Part model, mm, in its own coordinate system. Face numbers are marked on the shaded views. A direction names the side the tool comes from. Give positions to 0.01 mm unless a question says otherwise; leave off trailing zeros. Write each loop counter-clockwise with the first axis right and the second up, starting at its lowest first coordinate (ties: lowest second). Pieces come first, ordered by that corner, then holes. Notation, with made-up numbers: (-17, 85) - (25, 85) arc R23 cw to (25, 100) - close; hole circle Ø4 at (-13, 30.25). An arc over 180 degrees is marked (long way). Answer as a JSON object with one key per item and string values. Group by question number.
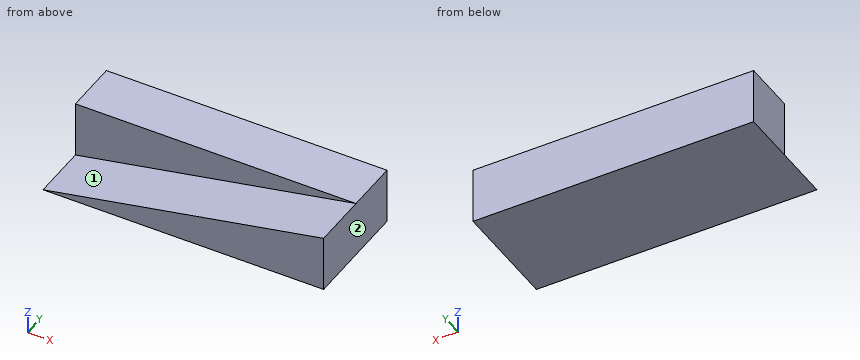
```python
from build123d import *

# Parameters (mm, degrees)
F0_W     = 126.529091
F0_H     = 49.704478
F1_DEPTH = 25.4
F3_DEPTH = 25.4


with BuildPart() as f1:
    # F0 (on Top) → F1 (new body)
    with BuildSketch(Plane.XY):
        with Locations((-4.691902, -11.49794)):
            Rectangle(F0_W, F0_H)
    extrude(amount=F1_DEPTH)

    # F2 (on face) → F3 (cut)
    with BuildSketch(Plane.XZ.offset(36.350179)):
        Polygon((-67.956448, 0), (58.572643, 25.4), (-67.956448, 25.4), align=None)
    extrude(amount=-F3_DEPTH, mode=Mode.SUBTRACT)


solid = f1.part
```
1) Saw through at B-B (z = 23.75). List the corners of the cut face in (x, y).
2) Drill centre lines: line 1 along Y through (x, z) = (-3.5, 18.75); line 2 along Z through (x, y) = (-31, -16); line 3 along Z through (x, y) = (33, -24). Where is each one in solid material? Low to high. Write a range as from..to.
3) Drop flat-ended pins along their axis: P1, Ø6, axis at x = -3.5, z = 22.5, coming from the -Y side; P2, Ø4, axis at x = -46.5, y = -26, coming from the +Z side. Give the stop position or say it passes through.
4) Which spindle directions (+Z, -Z, +X, -X, +Y, -Y) get a long thin tool onto all of the face, cutting with end or side? Do the marked faces 1 and 2. Say none if no direction does.
5) Saw through at C-C (x = 36). List the corners of the cut face in (y, z).
6) Saw through at A-A (y = -27). List the corners of the cut face in (x, z), and give its area (3 significant figures).
Checks:
{
 "1": {"outline": "(-67.96, -10.95) - (50.35, -10.95) - (50.35, -36.35) - (58.57, -36.35) - (58.57, 13.35) - (-67.96, 13.35) - close"},
 "2": {"line 1": "-10.95..13.35", "line 2": "0..7.42", "line 3": "0..20.27"},
 "3": {"P1": "y = -10.95", "P2": "z = 4.71"},
 "4": {"face 1": "+Z, -X, -Y", "face 2": "+Z, -Z, +X, +Y, -Y"},
 "5": {"outline": "(-36.35, 0) - (13.35, 0) - (13.35, 25.4) - (-10.95, 25.4) - (-10.95, 20.87) - (-36.35, 20.87) - close"},
 "6": {"outline": "(-67.96, 0) - (58.57, 0) - (58.57, 25.4) - close", "area": "1,610 mm2"}
}
